Design review of the part built by this model. Coordinates are the model's own, in mm. A direction names the side the tool comes from. Coordinates: 2 decimals unless noted, no trailing zeros. Loops run counter-clockwise (first coordinate to the right, second up) from the corner with the lowest first, then second, coordinate; pieces in that order, holes last.
from build123d import *

# Parameters (mm, degrees)
F0_R      = 30
F1_DEPTH  = 2
F2_W      = 2
F2_H      = 10
F3_DEPTH  = 25
F4_COUNT  = 3
F3_FACE_W = 2
F3_FACE_H = 10
F5_DEPTH  = 25
F6_DEPTH  = 25


with BuildPart() as f1:
    # F0 (on Top) → F1 (new body)
    with BuildSketch(Plane.XY):
        Circle(F0_R)
    extrude(amount=F1_DEPTH)

    # F4_face (on face) + F3_face (on face) → F5 (cut)
    with BuildSketch(Plane(origin=(10.4850735515, -18.1606801124, 2), x_dir=(1, 0, 0), z_dir=(0, 0, -1))):
        Polygon((-3.8301270189, 3.3660254038), (-4.8301270189, 1.6339745962), (3.8301270189, -3.3660254038), (4.8301270189, -1.6339745962), align=None)
        Polygon((4.8301270189, -34.6873856285), (3.8301270189, -32.9553348209), (-4.8301270189, -37.9553348209), (-3.8301270189, -39.6873856285), align=None)
    with BuildSketch(Plane(origin=(-20.9701471031, 0, 2), x_dir=(1, 0, 0), z_dir=(0, 0, -1))):
        Rectangle(F3_FACE_W, F3_FACE_H)
    extrude(amount=F5_DEPTH, mode=Mode.SUBTRACT)


with BuildPart() as f3:
    # F2 (on face) → F3 (new body)
    with BuildSketch(Plane.XY.offset(2)):
        with Locations((-20.9701471031, 0)):
            Rectangle(F2_W, F2_H)
    extrude(amount=F3_DEPTH)


with BuildPart() as f4_1:
    # F4: instance of F3
    add(f3.part.rotate(Axis((0, 0, 0), (0, 0, -1)), 1 * 360 / F4_COUNT))


with BuildPart() as f4_2:
    # F4: instance of F3
    add(f3.part.rotate(Axis((0, 0, 0), (0, 0, -1)), 2 * 360 / F4_COUNT))


with BuildPart() as f6_tool:
    # F3_face (on face) + F4_face (on face) → F6 (new body)
    with BuildSketch(Plane(origin=(-20.9701471031, 0, 2), x_dir=(1, 0, 0), z_dir=(0, 0, -1))):
        Rectangle(F3_FACE_W, F3_FACE_H)
    with BuildSketch(Plane(origin=(10.4850735515, -18.1606801124, 2), x_dir=(1, 0, 0), z_dir=(0, 0, -1))):
        Polygon((4.8301270189, -34.6873856285), (3.8301270189, -32.9553348209), (-4.8301270189, -37.9553348209), (-3.8301270189, -39.6873856285), align=None)
        Polygon((-3.8301270189, 3.3660254038), (-4.8301270189, 1.6339745962), (3.8301270189, -3.3660254038), (4.8301270189, -1.6339745962), align=None)
    extrude(amount=-F6_DEPTH)


with BuildPart() as f3_1:
    add(f3.part)

    # F6: cut by f6_tool
    add(f6_tool.part, mode=Mode.SUBTRACT)


with BuildPart() as f4_1_1:
    add(f4_1.part)

    # F6: cut by f6_tool
    add(f6_tool.part, mode=Mode.SUBTRACT)


with BuildPart() as f4_2_1:
    add(f4_2.part)

    # F6: cut by f6_tool
    add(f6_tool.part, mode=Mode.SUBTRACT)


solid = f1.part
Q1. Take a section at B-B, the plane z = 1.65. Write out the cut boundary in (x, y), then the cut area to 3 significant figures.
Q2. Clearance check with flat-ended pins moving along their axes: pin 1 Ø3 at (x, y) = (5.5, -18.5) entering from -Z; pin 2 Ø1 at (y, z) = (-11, 1.5) entering from -X; pin 3 Ø0.6 at (x, z) = (-20.5, 1) entering from +Y; pin 4 Ø1 at (y, z) = (-1.5, 1) entering from -X. State where each tip first meets the part, or that it passes through.
Q3. Take a section at C-C, the plane x = 9. Write out the cut boundary in (y, z), then the cut area to 3 significant figures.
Q4. Machinability: for faces 5 (the flat face through (-21, -5, 1)), 6 (the flat face through (0, 0, 0)), which of the approach directions +Z, -Z, +X, -X, +Y, -Y give a long, thin tool a straight path to every point of the face, cutting with its end or side? Answer none if there is none.
Q5. For line 1 (Y direction, x = 14, z = 1.15); line 2 (Y direction, x = 8, z = 1.25); line 3 (X direction, y = -21, z = 0.35), list the stretches that pass through material, from the lowest coordinate up.
Q6. Take a section at A-A, the plane y = 0. Write out the cut boundary in (x, z).
Q7. The part is to be moulded in two halves that separate along X. For faces 1 (the flat face through (0, 0, 2)), 2 (the flat face through (14.82, 15.67, 1.01)), 3 (the flat face through (6.15, 20.65, 1.01)), 4 (the cylindrical face through (-29.97, 1.32, 0.99)), say which applies: pulls with the +X half, pulls with the -X half, needs draft (parallel to the pull), parting line crosses it, or undercut.
Q8. Take a section at D-D, the plane x = -19. Write out the cut boundary in (y, z).
Entries:
1. outline: circle Ø60 at (0, 0); hole (-21.97, -5) - (-19.97, -5) - (-19.97, 5) - (-21.97, 5) - close; hole (5.65, -19.79) - (6.65, -21.53) - (15.32, -16.53) - (14.32, -14.79) - close; hole (5.65, 19.79) - (14.32, 14.79) - (15.32, 16.53) - (6.65, 21.53) - close
1. area: 2,770 mm2
2. pin 1: stops at z = 0
2. pin 2: stops at x = -28.1
2. pin 3: stops at y = 22.18
2. pin 4: stops at x = -29.98
3. outline: (-28.62, 0) - (-20.17, 0) - (-20.17, 2) - (-28.62, 2) - close; (-17.86, 0) - (17.86, 0) - (17.86, 2) - (-17.86, 2) - close; (20.17, 0) - (28.62, 0) - (28.62, 2) - (20.17, 2) - close
3. area: 105 mm2
4. face 5: +Z, -Z
4. face 6: -Z, +X, -X, +Y, -Y
5. line 1: y = -26.53 to -17.29, -14.98 to 14.98, 17.29 to 26.53
5. line 2: y = -28.91 to -20.75, -18.44 to 18.44, 20.75 to 28.91
5. line 3: x = -21.42 to 6.35, 7.57 to 21.42
6. outline: (-30, 0) - (-21.97, 0) - (-21.97, 2) - (-30, 2) - close; (-19.97, 0) - (30, 0) - (30, 2) - (-19.97, 2) - close
7. face 1: needs draft
7. face 2: undercut
7. face 3: undercut
7. face 4: parting line crosses it
8. outline: (-23.22, 0) - (23.22, 0) - (23.22, 2) - (-23.22, 2) - close
